Job drawing, mm, ordinate dimensions from the low corner. One solid piece. A direction names the side the tool comes from. Give positions to 0.01 mm unless a question says otherwise; leave off trailing zeros. Write each loop counter-clockwise with the first axis right and the second up, starting at its lowest first coordinate (ties: lowest second). Pieces come first, ordered by that corner, then holes. Notation, with made-up numbers: (-7, -0.75) - (1, -0.75) arc R21 cw to (1, 37.25) - close; hole circle Ø1 at (83.25, -20). An arc over 180 degrees is marked (long way). Answer as a JSON object with one key per item and string values.
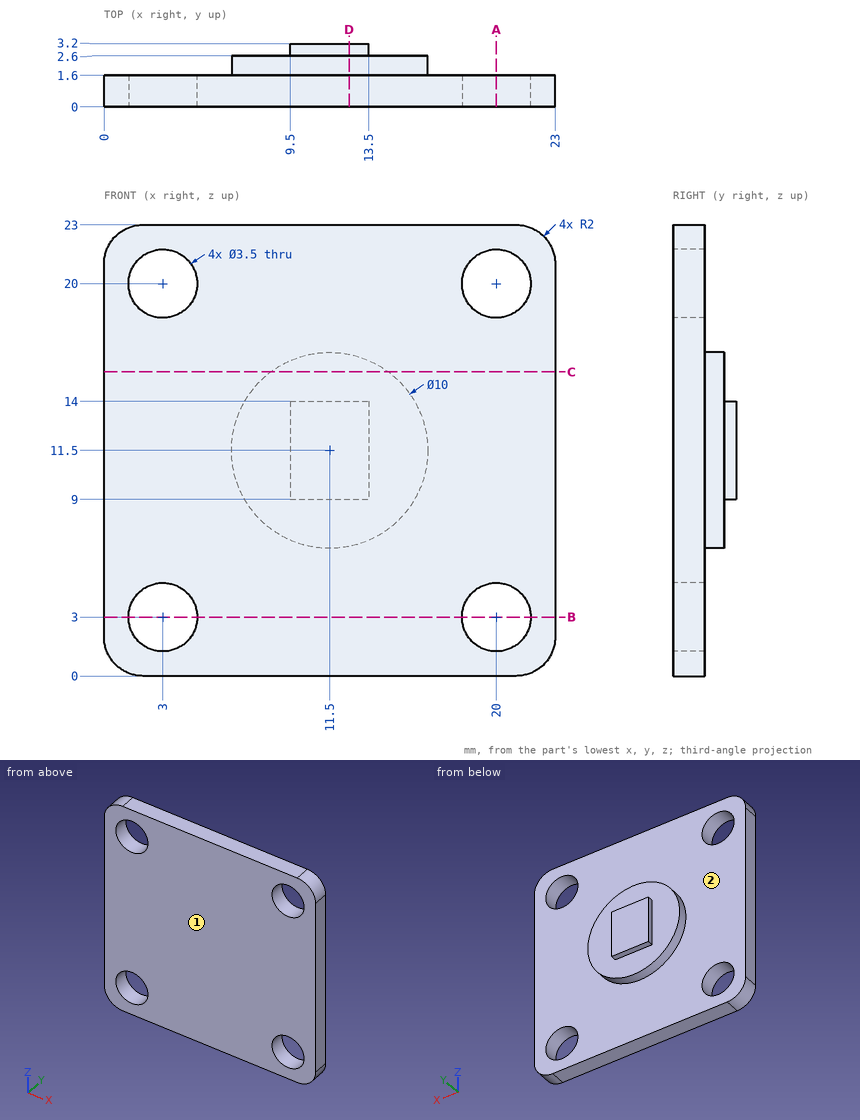
Item 1: Probe line 1 (Z direction, x = 20, y = 0.95); line 2 (Y direction, x = 1.75, z = 15.5). List the from-to ranges inside material, lowest first. Write a range as from..to.
Entries:
{"line 1": "0..1.25, 4.75..18.25, 21.75..23", "line 2": "0..1.6"}
Item 2: Cut at B-B (z = 3). Give the cut face in (x, y).
Entries:
{"outline": "(0, 0) - (1.25, 0) - (1.25, 1.6) - (0, 1.6) - close; (4.75, 0) - (18.25, 0) - (18.25, 1.6) - (4.75, 1.6) - close; (21.75, 0) - (23, 0) - (23, 1.6) - (21.75, 1.6) - close"}
Item 3: Flat gauge pins, fed straight in: P1, Ø1.5, axis at x = 10.5, y = 1.5, coming from the -Z side; P2, Ø5.5, axis at x = 20, z = 3, coming from the +Y side; P3, Ø0.5, axis at y = 3, z = 12, coming from the -X side. Where does each tip first touch, or does it go through?
Entries:
{"P1": "z = 0", "P2": "y = 1.6", "P3": "x = 9.5"}
Item 4: Cut at D-D (x = 12.5). Give the cut face in (y, z).
Entries:
{"outline": "(0, 0) - (1.6, 0) - (1.6, 6.6) - (2.6, 6.6) - (2.6, 9) - (3.2, 9) - (3.2, 14) - (2.6, 14) - (2.6, 16.4) - (1.6, 16.4) - (1.6, 23) - (0, 23) - close"}
Item 5: Cut at A-A (x = 20). Give the cut face in (y, z), and give its area (3 significant figures).
Entries:
{"outline": "(0, 0) - (1.6, 0) - (1.6, 1.25) - (0, 1.25) - close; (0, 4.75) - (1.6, 4.75) - (1.6, 18.25) - (0, 18.25) - close; (0, 21.75) - (1.6, 21.75) - (1.6, 23) - (0, 23) - close", "area": "25.6 mm2"}
Item 6: Which spindle directions (+Z, -Z, +X, -X, +Y, -Y) get a long thin tool onto all of the face, cutting with end or side? Do the marked faces 1 and 2. Say none if no direction does.
Entries:
{"face 1": "+Z, -Z, +X, -X, -Y", "face 2": "+Y"}
Item 7: Cut at C-C (z = 15.5). Give the cut face in (x, y), and give its area (3 significant figures).
Entries:
{"outline": "(0, 0) - (23, 0) - (23, 1.6) - (14.5, 1.6) - (14.5, 2.6) - (8.5, 2.6) - (8.5, 1.6) - (0, 1.6) - close", "area": "42.8 mm2"}
